Autodesk Fusion 360 part; units mm, degrees
sketch "Sketch9" plane through (0, 0, 0) normal (0, 0, 1) x (1, 0, 0)
  line L0 (-137.7795, 113.4984) -> (116.2205, 113.4984)
  line L1 (-137.7795, 113.4984) -> (-137.7795, -140.5016)
  line L2 (-137.7795, -140.5016) -> (116.2205, -140.5016)
  line L3 (116.2205, 113.4984) -> (116.2205, -140.5016)
extrude "Extrude2" add sketch "Sketch9" along normal blind 254
shell "Shell2" thickness 25.4 removed faces 1 at (-53.1129, -55.835, 0)
Input: part model. Units: mm. Frame: model coordinates. A direction names the side the tool comes from. Coordinates: 2 decimals unless noted, no trailing zeros. Loops run counter-clockwise (first coordinate to the right, second up) from the corner with the lowest first, then second, coordinate; pieces in that order, holes last.
Q1. Contact query for a flat-ended pin moving along its axis: pin 1 (10 mm diameter, centred on x = -8.5, y = 40.5, fed in from -Z). Output: stop coordinate, or through.
Results are:
pin 1: stops at z = 228.6
Q2. Section C-C, the plane x = 65. Return the cut outline in (y, z), and give its area (3 significant figures).
Results are:
outline: (-140.5, 0) - (-115.1, 0) - (-115.1, 228.6) - (88.1, 228.6) - (88.1, 0) - (113.5, 0) - (113.5, 254) - (-140.5, 254) - close
area: 18,100 mm2
Q3. Section B-B, the plane y = 42. Return the cut outline in (x, z), and give its area (3 significant figures).
Results are:
outline: (-137.78, 0) - (-112.38, 0) - (-112.38, 228.6) - (90.82, 228.6) - (90.82, 0) - (116.22, 0) - (116.22, 254) - (-137.78, 254) - close
area: 18,100 mm2
Q4. Set-up query: faces 1 (the flat face through (-13, -12, 254)), 2 (the flat face through (90.82, -12, 113)). Return all of +Z, -Z, +X, -X, +Y, -Y with unobstructed straight access to the full face (end or side cutting, diameter ignored); none if empty.
Results are:
face 1: +Z, +X, -X, +Y, -Y
face 2: -Z
Q5. Section A-A, the plane z = 166. Return the cut outline in (x, y), and give its area (3 significant figures).
Results are:
outline: (-137.78, -140.5) - (116.22, -140.5) - (116.22, 113.5) - (-137.78, 113.5) - close; hole (-112.38, -115.1) - (90.82, -115.1) - (90.82, 88.1) - (-112.38, 88.1) - close
area: 23,200 mm2
Q6. Mould query, pull axis Y, two halves, no side actions, for faces 3 (the flat face through (-13, 113.498, 125)), 4 (the flat face through (-112.38, -12, 113)), 5 (the flat face through (-13, -140.502, 125)). Classes: +Y half, -Y half, draft (parallel to the pull), parting line (faces both ways), or undercut.
Results are:
face 3: +Y half
face 4: undercut
face 5: -Y half
Q7. Line query: line 1 along Y through (x, z) = (-107, 126); line 2 along X through (y, z) = (-100, 161); line 3 along Z through (x, y) = (13, 59.5). Output: solid intervals per line, ascending.
Results are:
line 1: y = -140.5 to -115.1, 88.1 to 113.5
line 2: x = -137.78 to -112.38, 90.82 to 116.22
line 3: z = 228.6 to 254
